The model under review builds one solid part; all positions refer to its coordinate system, in mm. Coordinates: 2 decimals unless noted, no trailing zeros. Order: outer loops, then holes, each group sorted by start corner. A loop starts at its lowest first (then second) coordinate and runs counter-clockwise, first axis right, second up. Notation, with made-up numbers: M 6.5,57.5 L 48.5,57.5 A13 cw 48.5,66.5 Z; hole C 84,66.5 d4. An arc over 180 degrees is marked long. Write each question's results on one line, items separated by ' | '.
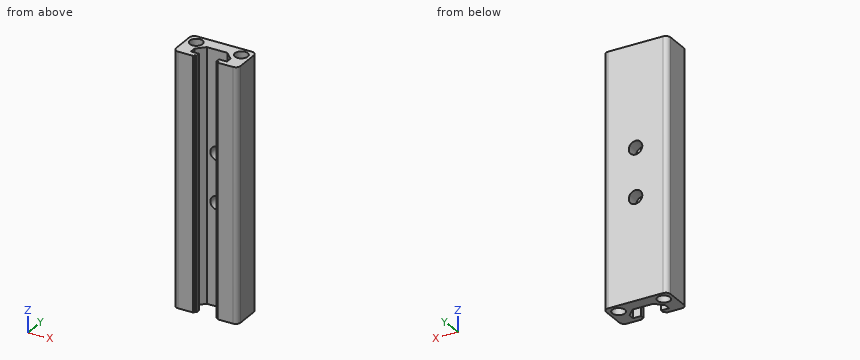
from build123d import *

# Parameters (mm, degrees)
SKETCH_1_R               = 2
EXTRUDE_1_DEPTH          = 39
CUT_EXTRUDE_1_DEPTH      = 42.484937025
CUT_EXTRUDE_1_DEPTH_BACK = 42.484937025
SKETCH_2_R               = 2.1


with BuildPart() as part:
    # 草图1 → 凸台-拉伸1 (new, symmetric)
    with BuildSketch(Plane.XY):
        with BuildLine():
            Line((-8.5, 0), (-3.95, 0))
            ThreePointArc((-3.95, 0), (-3.737867966, 0.087867966), (-3.65, 0.3))
            Line((-3.65, 0.3), (-3.65, 0.6))
            Line((-3.65, 0.6), (-3.1, 0.6))
            Line((-3.1, 0.6), (-3.1, 1.8))
            Line((-3.1, 1.8), (-5.6, 1.8))
            Line((-5.6, 1.8), (-5.6, 3.692893219))
            Line((-5.6, 3.692893219), (-3.192893219, 6.1))
            Line((-3.192893219, 6.1), (3.192893219, 6.1))
            Line((3.192893219, 6.1), (5.6, 3.692893219))
            Line((5.6, 3.692893219), (5.6, 1.8))
            Line((5.6, 1.8), (3.1, 1.8))
            Line((3.1, 1.8), (3.1, 0.6))
            Line((3.1, 0.6), (3.65, 0.6))
            Line((3.65, 0.6), (3.65, 0.3))
            ThreePointArc((3.65, 0.3), (3.737867966, 0.087867966), (3.95, 0))
            Line((3.95, 0), (8.5, 0))
            ThreePointArc((8.5, 0), (9.560660172, 0.439339828), (10, 1.5))
            Line((10, 1.5), (10, 8.5))
            ThreePointArc((10, 8.5), (9.560660172, 9.560660172), (8.5, 10))
            Line((8.5, 10), (-8.5, 10))
            ThreePointArc((-8.5, 10), (-9.560660172, 9.560660172), (-10, 8.5))
            Line((-10, 8.5), (-10, 1.5))
            ThreePointArc((-10, 1.5), (-9.560660172, 0.439339828), (-8.5, 0))
        make_face()
        with Locations((-7, 7)):
            Circle(SKETCH_1_R, mode=Mode.SUBTRACT)
        with Locations(Location((7, 7, 0), (0, 0, 180))):
            Circle(SKETCH_1_R, mode=Mode.SUBTRACT)
    extrude(amount=EXTRUDE_1_DEPTH, both=True)

    # 草图2 → 切除-拉伸1 (cut, two sides: drawn at the far end of the back side and taken through both)
    with BuildSketch(Plane(origin=(0, 10, 0), x_dir=(1, 0, 0), z_dir=(0, 1, 0)).offset(-CUT_EXTRUDE_1_DEPTH_BACK)):
        with Locations(Location((0, 7.5, 0), (0, 0, 270))):
            Circle(SKETCH_2_R)
        with Locations(Location((0, -7.5, 0), (0, 0, 270))):
            Circle(SKETCH_2_R)
    extrude(amount=CUT_EXTRUDE_1_DEPTH + CUT_EXTRUDE_1_DEPTH_BACK, mode=Mode.SUBTRACT)


solid = part.part
1) For pin 1 (1.9 mm diameter, centred on x = 1, z = -9.5, fed in from -Y); pin 2 (3.5 mm diameter, centred on x = -7, y = 7, fed in from -Z); pin 3 (6.5 mm diameter, centred on x = 0, z = -7.5, fed in from -Y), all flat-tipped, find the tip position at first contact; note any pin that passes through.
Solutions:
pin 1: y = 6.1 | pin 2: through | pin 3: y = 0.6
2) Take a section at D-D on z = 14. State the section outline as (x, y) points.
Solutions:
outline: M -10,1.5 A1.5 ccw -8.5,0 L -3.95,0 A0.3 ccw -3.65,0.3 L -3.65,0.6 L -3.1,0.6 L -3.1,1.8 L -5.6,1.8 L -5.6,3.69 L -3.19,6.1 L 3.19,6.1 L 5.6,3.69 L 5.6,1.8 L 3.1,1.8 L 3.1,0.6 L 3.65,0.6 L 3.65,0.3 A0.3 ccw 3.95,0 L 8.5,0 A1.5 ccw 10,1.5 L 10,8.5 A1.5 ccw 8.5,10 L -8.5,10 A1.5 ccw -10,8.5 Z; hole C -7,7 d4; hole C 7,7 d4
3) Take a section at C-C on x = 0. State the section outline as (y, z) points.
Solutions:
outline: M 6.1,-39 L 10,-39 L 10,-9.6 L 6.1,-9.6 Z; M 6.1,-5.4 L 10,-5.4 L 10,5.4 L 6.1,5.4 Z; M 6.1,9.6 L 10,9.6 L 10,39 L 6.1,39 Z
4) To check wall thickness, follow line 1 along Z through (x, y) = (0, 8.6); line 2 along X through (y, z) = (2.75, 7.5); line 3 along X through (y, z) = (8.6, -7.5). State the ranges of each line that lie inside material, in increasing order.
Solutions:
line 1: -39 to -9.6, -5.4 to 5.4, 9.6 to 39 | line 2: -10 to -5.6, 5.6 to 10 | line 3: -10 to -8.2, -5.8 to -2.1, 2.1 to 5.8, 8.2 to 10
5) Take a section at B-B on y = 7.75. State the section outline as (x, z) points.
Solutions:
outline: M -10,-39 L -8.85,-39 L -8.85,39 L -10,39 Z; M -5.15,-39 L 5.15,-39 L 5.15,39 L -5.15,39 Z; M 8.85,-39 L 10,-39 L 10,39 L 8.85,39 Z; hole C 0,-7.5 d4.2; hole C 0,7.5 d4.2
6) Take a section at A-A on z = -7.5. Count the separate pieces of the cut face and the enclosed holes in it, plus the area to 3 significant figures.
Solutions:
separate pieces: 2 | enclosed holes: 2 | area: 102 mm2
